```python
from build123d import *

# Parameters (mm, degrees)
F0_R     = 8.483319
F0_R_2   = 2.5
F1_DEPTH = 3.81


with BuildPart() as f1:
    # F0 (on Top) → F1 (new body)
    with BuildSketch(Plane.XY):
        Polygon((-32.063336, -31.690658), (-36.740027, -35.088473), (-20.701093, -40.047722), (-24.098908, -44.724413), (-7.312483, -44.484637), (-9.098819, -49.982417), (6.791925, -44.567085), (6.791925, -50.347793), (20.231491, -40.286997), (22.017828, -45.784776), (31.690658, -32.063336), (35.088473, -36.740027), (40.047722, -20.701093), (44.724413, -24.098908), (44.484637, -7.312483), (49.982417, -9.098819), (44.567085, 6.791925), (50.347793, 6.791925), (40.286997, 20.231491), (45.784776, 22.017828), (32.063336, 31.690658), (36.740027, 35.088473), (20.701093, 40.047722), (24.098908, 44.724413), (7.312483, 44.484637), (9.098819, 49.982417), (-6.791925, 44.567085), (-6.791925, 50.347793), (-20.231491, 40.286997), (-22.017828, 45.784776), (-31.690658, 32.063336), (-35.088473, 36.740027), (-40.047722, 20.701093), (-39.915663, 20.212912), (-44.716039, 23.512671), (-44.484637, 7.312483), (-49.982417, 9.098819), (-44.567085, -6.791925), (-50.347793, -6.791925), (-40.286997, -20.231491), (-45.784776, -22.017828), align=None)
        Circle(F0_R, mode=Mode.SUBTRACT)
        Circle(F0_R)
        Circle(F0_R_2, mode=Mode.SUBTRACT)
    extrude(amount=F1_DEPTH)


solid = f1.part
```
Input: part model. Units: mm. Frame: model coordinates. A direction names the side the tool comes from. Round coordinates to 2 decimals unless told otherwise and drop trailing zeros. Write each loop counter-clockwise with the first axis right and the second up, starting at its lowest first coordinate (ties: lowest second). Pieces come first, ordered by that corner, then holes. Notation, with made-up numbers: (-4.5, 14.25) - (34.5, 14.25) arc R19 cw to (34.5, 21.25) - close; hole circle Ø1 at (40, 14.25). An arc over 180 degrees is marked (long way). Write item = value, one per line.
(1) Section query C-C on x = -29. Output: boundary loops of the cut face in (y, z), then the cut area to 3 significant figures.
Geometry check:
outline = (-37.48, 0) - (35.88, 0) - (35.88, 3.81) - (-37.48, 3.81) - close
area = 280 mm^2
(2) Section query D-D on y = -38. Output: boundary loops of the cut face in (x, z).
Geometry check:
outline = (-27.32, 0) - (27.51, 0) - (27.51, 3.81) - (-27.32, 3.81) - close
(3) Contact query for flat-ended pins moving along their axis: pin 1 Ø1 at (x, z) = (3, 2.5) entering from -Y; pin 2 Ø1.9 at (x, z) = (48, 2) entering from -Y; pin 3 Ø2 at (y, z) = (34.5, 1) entering from -X. Output: stop coordinate, or through.
Geometry check:
pin_1 = -46.03
pin_2 = -8.76
pin_3 = -36.09
(4) Pull-direction query (X, two-part tool) for faces 6 (the flat face through (6.792, -47, 2)), 7 (the flat face through (34.369, 33.366, 1.878)), 8 (the flat face through (-47.31, 1.26, 1.88)); classes: +X half, -X half, draft (parallel to the pull), parting line (faces both ways), or undercut.
Geometry check:
face_6 = undercut
face_7 = +X half
face_8 = -X half
(5) Section query A-A on x = 0. Output: boundary loops of the cut face in (y, z), then the cut area to 3 significant figures.
Geometry check:
outline = (-46.88, 0) - (-2.5, 0) - (-2.5, 3.81) - (-46.88, 3.81) - close; (2.5, 0) - (46.88, 0) - (46.88, 3.81) - (2.5, 3.81) - close
area = 338 mm^2
(6) Material intervals for probe 1 along Y at (x, z) = (0, 2.3); probe 2 along Y at (x, z) = (-35, 2.15); probe 3 along X at (y, z) = (-43, 2), sorted ascending.
Geometry check:
probe_1 = -46.88 to -2.5, 2.5 to 46.88
probe_2 = -35.63 to -33.82, -29.62 to 36.62
probe_3 = -22.85 to 16.61, 21.11 to 23.98
(7) Access query for faces 1 (the flat face through (47, 6.792, 2)), 2 (the cylindrical face through (-0.54, -2.44, 1.88)), 3 (the flat face through (10, 1, 0)), 4 (the flat face through (-26.8, 39, 1.9)), 5 (the flat face through (-47, -6.792, 2)). Directions: +Z, -Z, +X, -X, +Y, -Y. A direction counts if a zero-diameter tool reaches every point of the face in a straight line with its end or side. Return the directions, or none.
Geometry check:
face_1 = +Z, -Z, +X
face_2 = +Z, -Z
face_3 = -Z, +X, -X, +Y, -Y
face_4 = +Z, -Z, +Y
face_5 = +Z, -Z, -X
